The model under review builds one solid part; all positions refer to its coordinate system, in mm. Face numbers are marked on the shaded views. Give positions to 0.01 mm unless a question says otherwise; leave off trailing zeros. Order: outer loops, then holes, each group sorted by start corner. A loop starts at its lowest first (then second) coordinate and runs counter-clockwise, first axis right, second up. Notation, with made-up numbers: (62.5, 39) - (95.5, 39) arc R16 ccw to (95.5, 44) - close; hole circle Ø2 at (1, -27.75). An arc over 180 degrees is marked (long way). Use CSV: the item, a comma, the result in double quotes. Start each with the question number.
1. For pin 1 (5.5 mm diameter, centred on y = 34, z = 20.5, fed in from -X); pin 2 (7.5 mm diameter, centred on x = -222.5, z = 23.5, fed in from +Y); pin 3 (9 mm diameter, centred on y = 33.5, z = 13, fed in from +X), all flat-tipped, find the tip position at first contact; note any pin that passes through.
2. Take a section at A-A, the plane x = -73. State the section outline as (y, z) points.
3. Draft analysis for pull direction Z (two halves, no side actions). For the marked faces 1, 2 and 3, state which applies: released by +Z, released by -Z, zero draft, split by the parting line, or undercut.
4. To check wall thickness, follow line 1 (Y direction, x = -184, z = 38); line 2 (Y direction, x = -299, z = 21.5). State the ranges of each line that lie inside material, in increasing order. Write a range as [from, to].
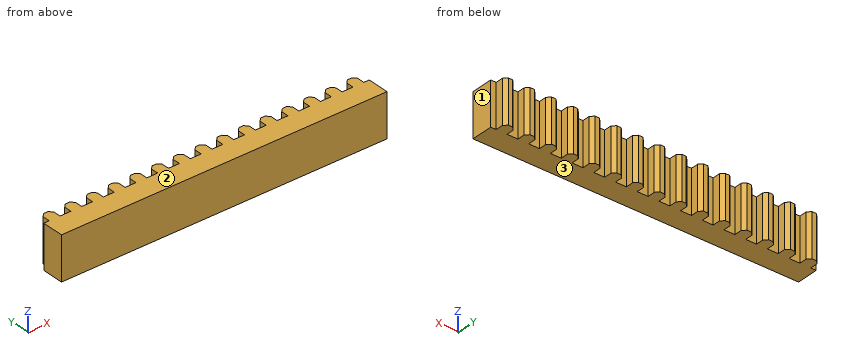
```python
from build123d import *

# Parameters (mm, degrees)
SKETCH1_W           = 762
SKETCH1_H           = 50.8
BOSS_EXTRUDE1_DEPTH = 50.8
SKETCH2_W           = 25.4
SKETCH2_H           = 25.363561455
BOSS_EXTRUDE2_DEPTH = 101.6
CHAMFER1_SIZE       = 7.62


with BuildPart() as part:
    # Sketch1 → Boss-Extrude1 (new body, symmetric)
    with BuildSketch(Plane.XY):
        Rectangle(SKETCH1_W, SKETCH1_H)
    extrude(amount=BOSS_EXTRUDE1_DEPTH, both=True)

    # Sketch2 → Boss-Extrude2 (add, through all)
    with BuildSketch(Plane.XY.offset(50.8)):
        with Locations((-254, 38.081780728)):
            Rectangle(SKETCH2_W, SKETCH2_H)
        with Locations((355.6, 38.081780728)):
            Rectangle(SKETCH2_W, SKETCH2_H)
        with Locations((0, 38.081780728)):
            Rectangle(SKETCH2_W, SKETCH2_H)
        with Locations((50.8, 38.081780728)):
            Rectangle(SKETCH2_W, SKETCH2_H)
        with Locations((101.6, 38.081780728)):
            Rectangle(SKETCH2_W, SKETCH2_H)
        with Locations((152.4, 38.081780728)):
            Rectangle(SKETCH2_W, SKETCH2_H)
        with Locations((203.2, 38.081780728)):
            Rectangle(SKETCH2_W, SKETCH2_H)
        with Locations((254, 38.081780728)):
            Rectangle(SKETCH2_W, SKETCH2_H)
        with Locations((304.8, 38.081780728)):
            Rectangle(SKETCH2_W, SKETCH2_H)
        with Locations((-50.8, 38.081780728)):
            Rectangle(SKETCH2_W, SKETCH2_H)
        with Locations((-101.6, 38.081780728)):
            Rectangle(SKETCH2_W, SKETCH2_H)
        with Locations((-152.4, 38.081780728)):
            Rectangle(SKETCH2_W, SKETCH2_H)
        with Locations((-203.2, 38.081780728)):
            Rectangle(SKETCH2_W, SKETCH2_H)
        with Locations((-304.8, 38.081780728)):
            Rectangle(SKETCH2_W, SKETCH2_H)
        with Locations((-355.6, 38.081780728)):
            Rectangle(SKETCH2_W, SKETCH2_H)
    extrude(amount=-BOSS_EXTRUDE2_DEPTH)

    # Chamfer1
    chamfer1_edges = [part.edges().sort_by_distance(p)[0] for p in [
        (-368.3, 50.763561455, 0),
        (-317.5, 50.763561455, 0),
        (-266.7, 50.763561455, 0),
        (-215.9, 50.763561455, 0),
        (-165.1, 50.763561455, 0),
        (-114.3, 50.763561455, 0),
        (-63.5, 50.763561455, 0),
        (-12.7, 50.763561455, 0),
        (38.1, 50.763561455, 0),
        (88.9, 50.763561455, 0),
        (139.7, 50.763561455, 0),
        (190.5, 50.763561455, 0),
        (241.3, 50.763561455, 0),
        (292.1, 50.763561455, 0),
        (342.9, 50.763561455, 0),
        (368.3, 50.763561455, 0),
        (317.5, 50.763561455, 0),
        (266.7, 50.763561455, 0),
        (215.9, 50.763561455, 0),
        (165.1, 50.763561455, 0),
        (114.3, 50.763561455, 0),
        (63.5, 50.763561455, 0),
        (12.7, 50.763561455, 0),
        (-38.1, 50.763561455, 0),
        (-88.9, 50.763561455, 0),
        (-139.7, 50.763561455, 0),
        (-190.5, 50.763561455, 0),
        (-241.3, 50.763561455, 0),
        (-342.9, 50.763561455, 0),
        (-292.1, 50.763561455, 0),
    ]]
    chamfer(chamfer1_edges, length=CHAMFER1_SIZE)


solid = part.part
```
Determined:
1,pin 1,"stops at x = -368.3"
1,pin 2,"stops at y = 25.4"
1,pin 3,"stops at x = 368.3"
2,outline,"(-25.4, -50.8) - (25.4, -50.8) - (25.4, 50.8) - (-25.4, 50.8) - close"
3,face 1,"zero draft"
3,face 2,"released by +Z"
3,face 3,"released by -Z"
4,line 1,"y = [-25.4, 25.4]"
4,line 2,"y = [-25.4, 50.04]"
